```python
from build123d import *

# Parameters (mm, degrees)
SKETCH1_R           = 16.5
BOSS_EXTRUDE1_DEPTH = 50
SKETCH2_R           = 17.5
CUT_EXTRUDE1_DEPTH  = 11
SKETCH3_R           = 2
CUT_EXTRUDE2_DEPTH  = 10
SCALE1_SCALE        = 1.771428571
BOSS_EXTRUDE2_START = -49.599999988
SKETCH4_R           = 29.228571421
SKETCH4_R_2         = 28.498571422
BOSS_EXTRUDE2_DEPTH = 49.599999988
CUT_EXTRUDE6_START  = -44.285714
SKETCH6_R           = 28.498571422
CUT_EXTRUDE6_DEPTH  = 19.285
CUT_EXTRUDE7_START  = 50.000714
SKETCH7_R           = 28.498571422
CUT_EXTRUDE7_DEPTH  = 19.285
SKETCH9_R           = 30.85
CUT_EXTRUDE8_DEPTH  = 23.8
SKETCH10_R          = 2
CUT_EXTRUDE9_DEPTH  = 50.00142855


with BuildPart() as part:
    # Sketch1 → Boss-Extrude1 (new body)
    with BuildSketch(Plane.XY):
        with BuildLine():
            Line((-15.968719423, 0), (15.968719423, 0))
            ThreePointArc((15.968719423, 0), (0, 51), (-15.968719423, 0))
        make_face()
        with Locations((0, 23)):
            Circle(SKETCH1_R, mode=Mode.SUBTRACT)
    extrude(amount=BOSS_EXTRUDE1_DEPTH)

    # Sketch2 → Cut-Extrude1 (cut)
    with BuildSketch(Plane.XY.offset(50)):
        with Locations((0, 23)):
            Circle(SKETCH2_R)
    cut_extrude1 = extrude(amount=-CUT_EXTRUDE1_DEPTH, mode=Mode.SUBTRACT)

    # Mirror1: Cut-Extrude1 across plane
    add(cut_extrude1.mirror(Plane.XY.offset(25)), mode=Mode.SUBTRACT)

    # Sketch3 → Cut-Extrude2 (cut)
    with BuildSketch(Plane(origin=(0, 0, 0), x_dir=(-1, 0, 0), z_dir=(0, 0, -1))):
        with Locations((0, 45.5)):
            Circle(SKETCH3_R)
        with Locations((-22.5, 23)):
            Circle(SKETCH3_R)
        with Locations((22.5, 23)):
            Circle(SKETCH3_R)
    cut_extrude2 = extrude(amount=-CUT_EXTRUDE2_DEPTH, mode=Mode.SUBTRACT)

    # Mirror2: Cut-Extrude2 across plane
    add(cut_extrude2.mirror(Plane.XY.offset(25)), mode=Mode.SUBTRACT)


with BuildPart() as part_1:
    # Scale1: scaled about (0, 24.810283146, 25)
    add(part.part.scale(SCALE1_SCALE).moved(Location((0, -19.139361273, -19.285714275))))

    # Sketch4 → Boss-Extrude2 (add)
    with BuildSketch(Plane.XY.offset(49.799999994).offset(BOSS_EXTRUDE2_START)):
        with Locations((0, 21.60349586)):
            Circle(SKETCH4_R)
        with Locations((0, 21.60349586)):
            Circle(SKETCH4_R_2, mode=Mode.SUBTRACT)
    extrude(amount=BOSS_EXTRUDE2_DEPTH)

    # Sketch6 → Cut-Extrude6 (cut)
    with BuildSketch(Plane.XY.offset(25).offset(CUT_EXTRUDE6_START)):
        with BuildLine():
            Line((-28.287445828, -19.139361273), (28.287445828, -19.139361273))
            ThreePointArc((28.287445828, -19.139361273), (0, 71.203495848), (-28.287445828, -19.139361273))
        make_face()
        with Locations((0, 21.60349586)):
            Circle(SKETCH6_R, mode=Mode.SUBTRACT)
    extrude(amount=CUT_EXTRUDE6_DEPTH, mode=Mode.SUBTRACT)

    # Sketch7 → Cut-Extrude7 (cut)
    with BuildSketch(Plane.XY.offset(CUT_EXTRUDE7_START)):
        with BuildLine():
            Line((-28.287445828, -19.139361273), (28.287445828, -19.139361273))
            ThreePointArc((28.287445828, -19.139361273), (0, 71.203495848), (-28.287445828, -19.139361273))
        make_face()
        with Locations((0, 21.60349586)):
            Circle(SKETCH7_R, mode=Mode.SUBTRACT)
    extrude(amount=CUT_EXTRUDE7_DEPTH, mode=Mode.SUBTRACT)

    # Sketch9 → Cut-Extrude8 (cut)
    with BuildSketch(Plane.XY.offset(50.000714275)):
        with Locations((0, 21.60349586)):
            Circle(SKETCH9_R)
    cut_extrude8 = extrude(amount=-CUT_EXTRUDE8_DEPTH, mode=Mode.SUBTRACT)

    # Mirror3: Cut-Extrude8 across plane
    add(cut_extrude8.mirror(Plane.XY.offset(25)), mode=Mode.SUBTRACT)

    # Sketch10 → Cut-Extrude9 (cut)
    with BuildSketch(Plane.XY.offset(50.000714275)):
        with Locations((0, 61.90349586)):
            Circle(SKETCH10_R)
        with Locations((-40.233402491, 23.919381004)):
            Circle(SKETCH10_R)
        with Locations((40.233400771, 23.919410876)):
            Circle(SKETCH10_R)
    extrude(amount=-CUT_EXTRUDE9_DEPTH, mode=Mode.SUBTRACT)


solid = part_1.part
```
Geometry: final body of the model. Coordinates: model frame, mm. A direction names the side the tool comes from. Coordinates: 2 decimals unless noted, no trailing zeros. Order: outer loops, then holes, each group sorted by start corner. A loop starts at its lowest first (then second) coordinate and runs counter-clockwise, first axis right, second up. Notation, with made-up numbers: M -8.75,8 L 47.25,8 A29 cw 47.25,34 Z; hole C 14.25,-8.5 d11. An arc over 180 degrees is marked long. Answer in a Markdown table with one row per item. Add a question column.
Q1. Line query: L1, parallel to Y at x = 0, z = 22; L2, parallel to Y at x = 0, z = 0.1; L3, parallel to Z at x = -29, y = 19. Output: solid intervals per line, ascending.
Q2. Section query D-D on z = 21.5. Return the cut outline in (x, y), and give its area (3 significant figures).
Q3. Mould query, pull axis Y, two halves, no side actions, for faces 1 (the cylindrical face through (0.923, 60.129, 25.35)), 2 (the flat face through (-23, 47, -0.001)), 3 (the flat face through (0, -19.139, 25)). Classes: released by +Y, released by -Y, zero draft, split by the parting line, or undercut.
Q4. Contact query for flat-ended pins moving along their axis: P1, Ø2.5, axis at x = -40.23, y = 23.92, coming from the +Z side; P2, Ø8, axis at y = 0, z = 24, coming from the -X side; P3, Ø12, axis at y = 37, z = 14, coming from the +X side; P4, Ø1, axis at x = -27, z = 24, coming from the +Y side. Output: stop coordinate, or through.
Q5. Section query C-C on x = 19. Return the cut outline in (y, z).
Q6. Section query A-A on x = 0. Return the cut outline in (y, z), and give its area (3 significant figures).
Q7. Reachability of faces 4 (the cylindrical face through (-4.02, 52.19, 38.17)), 5 (the cylindrical face through (-42.23, 24.01, 25.35)), 6 (the cylindrical face through (-4.02, 52.19, 11.83)) from +Z, -Z, +X, -X, +Y, -Y: full face, straight path, thin tool, end or side. Return the list, or none.
Q8. Section query B-B on y = 42.5. Return the cut outline in (x, z).
Completed:
| question | item | result |
|---|---|---|
| 1 | L1 | y = -19.14 to -9.25, 52.45 to 59.9, 63.9 to 71.2 |
| 1 | L2 | y = -19.14 to -9.4, 52.6 to 59.9, 63.9 to 71.2 |
| 1 | L3 | z = 23.8 to 26.2 |
| 2 | outline | M -28.29,-19.14 L 28.29,-19.14 A49.6 ccw long Z; hole C -40.23,23.92 d4; hole C 0,21.6 d61.7; hole C 0,61.9 d4; hole C 40.23,23.92 d4 |
| 2 | area | 4,360 mm2 |
| 3 | face 1 | undercut |
| 3 | face 2 | zero draft |
| 3 | face 3 | released by -Y |
| 4 | P1 | passes through |
| 4 | P2 | stops at x = -46.37 |
| 4 | P3 | stops at x = 48.7 |
| 4 | P4 | stops at y = 63.53 |
| 5 | outline | M -19.14,0 L -2.89,0 L -2.89,0.2 L -2.7,0.2 L -2.7,23.8 L 0.36,23.8 L 0.36,26.2 L -2.7,26.2 L -2.7,49.8 L -2.89,49.8 L -2.89,50 L -19.14,50 Z; M 42.84,23.8 L 45.91,23.8 L 45.91,0.2 L 46.1,0.2 L 46.1,0 L 67.42,0 L 67.42,50 L 46.1,50 L 46.1,49.8 L 45.91,49.8 L 45.91,26.2 L 42.84,26.2 Z |
| 6 | outline | M -19.14,0 L -9.4,0 L -9.4,0.2 L -9.25,0.2 L -9.25,23.8 L -6.9,23.8 L -6.9,26.2 L -9.25,26.2 L -9.25,49.8 L -9.4,49.8 L -9.4,50 L -19.14,50 Z; M 50.1,23.8 L 52.45,23.8 L 52.45,0.2 L 52.6,0.2 L 52.6,0 L 59.9,0 L 59.9,50 L 52.6,50 L 52.6,49.8 L 52.45,49.8 L 52.45,26.2 L 50.1,26.2 Z; M 63.9,0 L 71.2,0 L 71.2,50 L 63.9,50 Z |
| 6 | area | 1,240 mm2 |
| 7 | face 4 | +Z |
| 7 | face 5 | +Z, -Z |
| 7 | face 6 | -Z |
| 8 | outline | M -44.98,0 L -22.9,0 L -22.9,0.2 L -22.69,0.2 L -22.69,23.8 L -19.38,23.8 L -19.38,26.2 L -22.69,26.2 L -22.69,49.8 L -22.9,49.8 L -22.9,50 L -44.98,50 Z; M 19.38,23.8 L 22.69,23.8 L 22.69,0.2 L 22.9,0.2 L 22.9,0 L 44.98,0 L 44.98,50 L 22.9,50 L 22.9,49.8 L 22.69,49.8 L 22.69,26.2 L 19.38,26.2 Z |
